from build123d import *

# Parameters (mm, degrees)
BOSS_EXTRUDE1_DEPTH     = 5.5
SKETCH2_W               = 65
SKETCH2_H               = 25.5
BOSS_EXTRUDE2_DEPTH     = 5
SKETCH3_W               = 55
SKETCH3_H               = 25
BOSS_EXTRUDE3_DEPTH     = 5
SKETCH4_W               = 42
SKETCH4_H               = 55
BOSS_EXTRUDE4_DEPTH     = 5
BOSS_EXTRUDE6_DEPTH     = 7.5
BOSS_EXTRUDE7_DEPTH     = 42
SKETCH7_W               = 5
SKETCH7_H               = 29.5
BOSS_EXTRUDE8_DEPTH     = 5
SKETCH8_W               = 55
SKETCH8_H               = 20
CUT_EXTRUDE1_DEPTH      = 5
SKETCH9_R               = 2.5
SKETCH9_R_2             = 2
CUT_EXTRUDE2_DEPTH      = 98.155802709
SKETCH10_R              = 2
CUT_EXTRUDE3_DEPTH      = 91.21640649
CUT_EXTRUDE4_DEPTH      = 87.972696865
CUT_EXTRUDE4_DEPTH_BACK = 87.972696865
SKETCH11_R              = 1.75
SKETCH11_R_2            = 11
CHAMFER1_SIZE           = 5
SKETCH12_W              = 14
SKETCH12_H              = 5
CUT_EXTRUDE5_DEPTH      = 10


with BuildPart() as part:
    # Sketch1 → Boss-Extrude1 (new body)
    with BuildSketch(Plane.XY):
        Polygon((-40, 20), (-40, 0), (0, -25), (20, -25), (67, 0), (25, 0), (25, 20), align=None)
    extrude(amount=BOSS_EXTRUDE1_DEPTH)

    # Sketch2 → Boss-Extrude2 (add)
    with BuildSketch(Plane(origin=(0, 20, 0), x_dir=(1, 0, 0), z_dir=(0, 1, 0))):
        with Locations((-7.5, 7.25)):
            Rectangle(SKETCH2_W, SKETCH2_H)
    extrude(amount=BOSS_EXTRUDE2_DEPTH)

    # Sketch3 → Boss-Extrude3 (add)
    with BuildSketch(Plane(origin=(25, 0, 0), x_dir=(0, 0, -1), z_dir=(1, 0, 0))):
        with Locations((22, 12.5)):
            Rectangle(SKETCH3_W, SKETCH3_H)
    extrude(amount=BOSS_EXTRUDE3_DEPTH)

    # Sketch4 → Boss-Extrude4 (add)
    with BuildSketch(Plane(origin=(0, 0, 0), x_dir=(1, 0, 0), z_dir=(0, 1, 0))):
        with Locations((46, 22)):
            Rectangle(SKETCH4_W, SKETCH4_H)
    extrude(amount=BOSS_EXTRUDE4_DEPTH)

    # Sketch5 → Boss-Extrude6 (add)
    with BuildSketch(Plane(origin=(0, 0, 0), x_dir=(-1, 0, 0), z_dir=(0, 0, -1))):
        Polygon((-20, -25), (-20, 20), (-25, 20), (-25, 0), (-67, 0), align=None)
    extrude(amount=BOSS_EXTRUDE6_DEPTH)

    # Sketch6 → Boss-Extrude7 (add)
    with BuildSketch(Plane(origin=(0, 0, -7.5), x_dir=(-1, 0, 0), z_dir=(0, 0, -1))):
        Polygon((-25, 0), (-25, -22.340425532), (-20, -25), (-20, 20), (-25, 20), align=None)
    extrude(amount=BOSS_EXTRUDE7_DEPTH)

    # Sketch7 → Boss-Extrude8 (add)
    with BuildSketch(Plane(origin=(0, 20, 0), x_dir=(1, 0, 0), z_dir=(0, 1, 0))):
        with Locations((22.5, 34.75)):
            Rectangle(SKETCH7_W, SKETCH7_H)
    extrude(amount=BOSS_EXTRUDE8_DEPTH)

    # Sketch8 → Cut-Extrude1 (cut)
    with BuildSketch(Plane(origin=(30, 0, 0), x_dir=(0, 0, -1), z_dir=(1, 0, 0))):
        with Locations((22, 15)):
            Rectangle(SKETCH8_W, SKETCH8_H)
    extrude(amount=-CUT_EXTRUDE1_DEPTH, mode=Mode.SUBTRACT)

    # Sketch9 → Cut-Extrude2 (cut, through all)
    with BuildSketch(Plane(origin=(0, 25, 0), x_dir=(1, 0, 0), z_dir=(0, 1, 0))):
        with Locations(Location((10, 10, 0), (0, 0, 270))):
            Circle(SKETCH9_R)
        with Locations(Location((-33.5, 10, 0), (0, 0, 270))):
            Circle(SKETCH9_R_2)
        with Locations(Location((-20, 10, 0), (0, 0, 270))):
            Circle(SKETCH9_R_2)
        with Locations(Location((-6.5, 10, 0), (0, 0, 270))):
            Circle(SKETCH9_R_2)
    extrude(amount=-CUT_EXTRUDE2_DEPTH, mode=Mode.SUBTRACT)

    # Sketch10 → Cut-Extrude3 (cut, through all)
    with BuildSketch(Plane.XY.offset(5.5)):
        with Locations((-33.5, 10)):
            Circle(SKETCH10_R)
        with Locations((-20, 10)):
            Circle(SKETCH10_R)
        with Locations((-6.5, 10)):
            Circle(SKETCH10_R)
        with Locations((10, -18.5)):
            Circle(SKETCH10_R)
        with Locations((10, -7.833333333)):
            Circle(SKETCH10_R)
        with Locations((10, 2.833333333)):
            Circle(SKETCH10_R)
        with Locations((10, 13.5)):
            Circle(SKETCH10_R)
    extrude(amount=-CUT_EXTRUDE3_DEPTH, mode=Mode.SUBTRACT)

    # Sketch11 → Cut-Extrude4 (cut, two sides: drawn at the far end of the back side and taken through both)
    with BuildSketch(Plane.XZ.offset(-CUT_EXTRUDE4_DEPTH_BACK)):
        with Locations(Location((61.5, -44, 0), (0, 0, 90))):
            Circle(SKETCH11_R)
        with Locations(Location((61.5, -13, 0), (0, 0, 90))):
            Circle(SKETCH11_R)
        with Locations(Location((30.5, -13, 0), (0, 0, 90))):
            Circle(SKETCH11_R)
        with Locations(Location((30.5, -44, 0), (0, 0, 90))):
            Circle(SKETCH11_R)
        with Locations(Location((46, -28.5, 0), (0, 0, 90))):
            Circle(SKETCH11_R_2)
    extrude(amount=CUT_EXTRUDE4_DEPTH + CUT_EXTRUDE4_DEPTH_BACK, mode=Mode.SUBTRACT)

    # Chamfer1
    chamfer1_edges = [part.edges().sort_by_distance(p)[0] for p in [
        (67, 2.5, -49.5),
    ]]
    chamfer(chamfer1_edges, length=CHAMFER1_SIZE)

    # Sketch12 → Cut-Extrude5 (cut)
    with BuildSketch(Plane(origin=(25, 0, 0), x_dir=(0, 0, -1), z_dir=(1, 0, 0))):
        with Locations((28, 16.5)):
            Rectangle(SKETCH12_W, SKETCH12_H)
    extrude(amount=-CUT_EXTRUDE5_DEPTH, mode=Mode.SUBTRACT)


solid = part.part
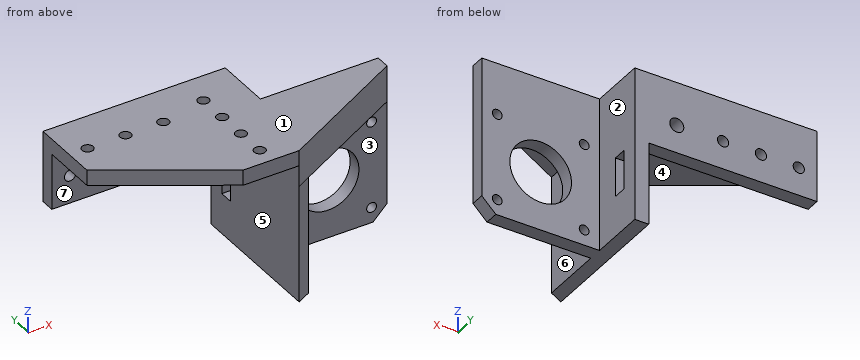
Could you check a few things on this model? Use its own coordinates, in mm. Face numbers are marked on the shaded views. A direction names the side the tool comes from. Give positions to 0.01 mm unless a question says otherwise; leave off trailing zeros. Order: outer loops, then holes, each group sorted by start corner. A loop starts at its lowest first (then second) coordinate and runs counter-clockwise, first axis right, second up.
Item 1: If we section it at B-B, the plane y = -18.5: Write out the boundary of the cut face in (x, z), plus the area to 3 significant figures.
Item 2: For the marked faces 1, 2, 3 and 4, which set-ups out of +Z, -Z, +X, -X, +Y, -Y let a thin tool reach every point of the face, with its end or its side?
Item 3: If we section it at A-A, the plane z = -10: Write out the boundary of the cut face in (x, y), plus the area to 3 significant figures.
Item 4: If we section it at D-D, the plane z = -23.5: Write out the boundary of the cut face in (x, y), plus the area to 3 significant figures.
Item 5: I need wall thicknesses on line 1 (Y direction, x = 10, z = 4); line 2 (X direction, y = 11.5, z = -33.5); line 3 (Z direction, x = 45.5, y = -1). Which ranges of each line are inside material? Lowest first, please.
Item 6: If we mould it in two halves opening along X, with no side actions, what happens to the marked faces 5, 6 and 7? For each: pulls with the +X half, pulls with the -X half, needs draft (parallel to the pull), parting line crosses it, or undercut.
Item 7: I'm going to push flat-ended pins straight in: pin 1 (4.5 mm diameter, centred on x = -33.5, y = 10, fed in from -Z); pin 2 (2 mm diameter, centred on y = -10.5, z = -35.5, fed in from -X); pin 3 (1 mm diameter, centred on y = -10.5, z = -16, fed in from +X); pin 4 (6.5 mm diameter, centred on x = -6.5, y = 10, fed in from +Z). Where does each tip first touch, or does it pass through?
Item 8: If we section it at C-C, the plane x = 46: Write out the boundary of the cut face in (y, z).
Values:
1. outline: (-10.4, 0) - (8, 0) - (8, 5.5) - (-10.4, 5.5) - close; (12, 0) - (20, 0) - (20, -49.5) - (25, -49.5) - (25, -7.5) - (32.22, -7.5) - (32.22, 5.5) - (12, 5.5) - close
1. area: 514 mm2
2. face 1: +Z, +X, -X, +Y, -Y
2. face 2: +Z, -Z, +X, +Y
2. face 3: -Z, +X, -Y
2. face 4: -Z, -X, -Y
3. outline: (-40, 20) - (-35.5, 20) - (-35.5, 25) - (-40, 25) - close; (-31.5, 20) - (-22, 20) - (-22, 25) - (-31.5, 25) - close; (-18, 20) - (-8.5, 20) - (-8.5, 25) - (-18, 25) - close; (-4.5, 20) - (7.5, 20) - (7.5, 25) - (-4.5, 25) - close; (12.5, 20) - (20, 20) - (20, -25) - (25, -22.34) - (25, 0) - (67, 0) - (67, 5) - (25, 5) - (25, 25) - (12.5, 25) - close
3. area: 668 mm2
4. outline: (20, -25) - (25, -22.34) - (25, 0) - (36.2, 0) - (36.2, 5) - (25, 5) - (25, 14) - (20, 14) - close; (20, 19) - (25, 19) - (25, 25) - (20, 25) - close; (55.8, 0) - (67, 0) - (67, 5) - (55.8, 5) - close
4. area: 330 mm2
5. line 1: y = -25 to -20.5, -16.5 to -9.83, -5.83 to 0.83, 4.83 to 11.5, 15.5 to 25
5. line 2: x = 20 to 25
5. line 3: z = -7.5 to 5.5
6. face 5: pulls with the -X half
6. face 6: pulls with the +X half
6. face 7: needs draft
7. pin 1: stops at z = 0
7. pin 2: stops at x = 20
7. pin 3: stops at x = 25
7. pin 4: stops at z = 5.5
8. outline: (-11.17, -7.5) - (0, -7.5) - (0, -17.5) - (5, -17.5) - (5, 5.5) - (-11.17, 5.5) - close; (0, -49.5) - (5, -49.5) - (5, -39.5) - (0, -39.5) - close
